Geometry check sheet. Reference: the model listing, model coordinates, mm. A direction names the side the tool comes from. Give positions to 0.01 mm unless a question says otherwise; leave off trailing zeros. Write each loop counter-clockwise with the first axis right and the second up, starting at its lowest first coordinate (ties: lowest second). Pieces come first, ordered by that corner, then holes. Notation, with made-up numbers: (37, 57.25) - (60, 57.25) arc R23 ccw to (60, 93.25) - close; hole circle Ø6 at (5.5, -4.75). An arc over 180 degrees is marked (long way). One line per question, with ' | ' between items. Start each with the question number.
Q1. Section check D-D on y = 2. Record the boundary of the cut face in (x, z), and give its area (3 significant figures).
Q2. Section check B-B on x = 172.5. Record the boundary of the cut face in (y, z).
Q3. Thickness scan on L1, parallel to X at y = -37.5, z = -74.5; L2, parallel to Z at x = 89, y = 19.5; L3, parallel to Z at x = -43, y = 19. Record the ranges inside material, lowest first. Write a range as [from, to].
Q4. Section check A-A on z = -41. Record the boundary of the cut face in (x, y).
Q5. Set-up check for faces 3 (the face through (-155.67, 36.47, -20.76)), 4 (the face through (179, 36, -74.982)), 5 (the face through (140.335, -20.881, -55.169)), 6 (the face through (-21, 37, -31.802)): record each of +Z, -Z, +X, -X, +Y, -Y from which the full face is reachable in a straight line by a thin tool's end or side.
Q6. Release check for a two-part mould opening along X. For faces 1 (the face through (-104.14, 36, -18)), 2 (the face through (3, 15, 0)) record: +X half, -X half, draft (parallel to the pull), parting line (faces both ways), or undercut.
Q7. Gauge pin test, flat ends, axial feed: P1, Ø1, axis at x = 5, z = -45, coming from the +Y side; P2, Ø9.5, axis at x = 173, z = -97.5, coming from the -Y side; P3, Ø1.5, axis at y = 32, z = -35.5, coming from the -X side; P4, Ø8.5, axis at y = -28.5, z = -69, coming from the -X side. Record the tip position at first contact, or that the pin passes through.
Q8. Section check C-C on x = -35.5. Record the boundary of the cut face in (y, z).
```python
from build123d import *

# Parameters (mm, degrees)
BOSS_EXTRUDE1_DEPTH                 = 111.76
SKETCH5_W                           = 304.8
SKETCH5_H                           = 25.4
CUT_EXTRUDE3_DEPTH                  = 101.6
CUT_EXTRUDE4_DEPTH                  = 227.288199427
CUT_EXTRUDE4_DEPTH_BACK             = 227.288199427
SKETCH3_W                           = 96.52
SKETCH3_H                           = 101.6
SKETCH3_W_2                         = 48.26
CUT_EXTRUDE5_REACH                  = 288.663
SKETCH6_W                           = 38.1
SKETCH6_H                           = 50.8
SKETCH7_W                           = 81.28
SKETCH7_H                           = 50.8
BOSS_EXTRUDE2_DEPTH                 = 5.08
SKETCH9_W                           = 5.08
SKETCH9_H                           = 95.25
BOSS_EXTRUDE3_DEPTH                 = 10.16
SKETCH10_W                          = 5.08
SKETCH10_H                          = 95.206439839
BOSS_EXTRUDE4_DEPTH                 = 10.16
CUT_EXTRUDE7_REACH                  = 208.854
FILLET1_R                           = 50.8
BOSS_EXTRUDE5_REACH                 = 208.854
CUT_EXTRUDE8_REACH                  = 248.593
CUT_EXTRUDE8_END_RADIUS             = 126.32098656
CUT_EXTRUDE8_DIRECTION_2_REACH      = 248.593
CUT_EXTRUDE8_DIRECTION_2_END_RADIUS = 126.32098656


with BuildPart() as part:
    # Sketch1 → Boss-Extrude1 (new body)
    with BuildSketch(Plane.XY):
        Polygon((-152.4, 62.23), (-152.4, -33.02), (0, -62.23), (152.4, -32.976439839), (152.4, 62.23), align=None)
    extrude(amount=-BOSS_EXTRUDE1_DEPTH)

    # Sketch5 → Cut-Extrude3 (cut)
    with BuildSketch(Plane.XY.offset(-5.08)):
        with Locations((0, -1.27)):
            Rectangle(SKETCH5_W, SKETCH5_H)
    extrude(amount=-CUT_EXTRUDE3_DEPTH, mode=Mode.SUBTRACT)

    # Sketch3 → Cut-Extrude4 (cut, two sides: drawn at the far end of the back side and taken through both)
    with BuildSketch(Plane(origin=(0, 62.23, 0), x_dir=(1, 0, 0), z_dir=(0, 1, 0)).offset(-CUT_EXTRUDE4_DEPTH_BACK)):
        with Locations((-50.8, 55.88)):
            Rectangle(SKETCH3_W, SKETCH3_H)
        with Locations((50.8, 55.88)):
            Rectangle(SKETCH3_W, SKETCH3_H)
        with Locations((-128.27, 55.88)):
            Rectangle(SKETCH3_W_2, SKETCH3_H)
        with Locations((128.27, 55.88)):
            Rectangle(SKETCH3_W_2, SKETCH3_H)
    extrude(amount=CUT_EXTRUDE4_DEPTH + CUT_EXTRUDE4_DEPTH_BACK, mode=Mode.SUBTRACT)

    # Cut-Extrude5: up to this face of the body (flat: up to its plane)
    cut_extrude5_end = Plane(part.part.faces().sort_by_distance((104.14, 36.83, -55.88))[0])
    # Sketch6 → Cut-Extrude5 (cut, up to the picked face)
    with BuildSketch(Plane.ZY.offset(104.14), mode=Mode.PRIVATE) as cut_extrude5_sk1:
        with Locations((-55.932057734, 36.83)):
            Rectangle(SKETCH6_W, SKETCH6_H)
    cut_extrude5_tool1 = split(extrude(cut_extrude5_sk1.sketch, amount=-CUT_EXTRUDE5_REACH, mode=Mode.PRIVATE), bisect_by=cut_extrude5_end, keep=Keep.BOTH, mode=Mode.PRIVATE)
    add(cut_extrude5_tool1.solids().sort_by(Axis((-104.14, 36.83, -55.932058), (1, 0, 0)))[0], mode=Mode.SUBTRACT)

    # Sketch7 → Boss-Extrude2 (add)
    with BuildSketch(Plane(origin=(0, 0, -36.882057734), x_dir=(-1, 0, 0), z_dir=(0, 0, -1))):
        with Locations((0, 36.83)):
            Rectangle(SKETCH7_W, SKETCH7_H)
        with Locations((101.6, 36.83)):
            Rectangle(SKETCH7_W, SKETCH7_H)
        with Locations((-101.6, 36.83)):
            Rectangle(SKETCH7_W, SKETCH7_H)
    boss_extrude2 = extrude(amount=-BOSS_EXTRUDE2_DEPTH)

    # Mirror1: Boss-Extrude2 across plane
    add(boss_extrude2.mirror(Plane(origin=(0, 0, -55.932057734), x_dir=(1, 0, 0), z_dir=(0, 0, -1))))

    # Sketch9 → Boss-Extrude3 (add)
    with BuildSketch(Plane.ZY.offset(152.4)):
        with Locations((-109.22, 14.605)):
            Rectangle(SKETCH9_W, SKETCH9_H)
        with Locations((-2.54, 14.605)):
            Rectangle(SKETCH9_W, SKETCH9_H)
    extrude(amount=BOSS_EXTRUDE3_DEPTH)

    # Sketch10 → Boss-Extrude4 (add)
    with BuildSketch(Plane(origin=(152.4, 0, 0), x_dir=(0, 0, -1), z_dir=(1, 0, 0))):
        with Locations((2.54, 14.626780081)):
            Rectangle(SKETCH10_W, SKETCH10_H)
        with Locations((109.22, 14.626780081)):
            Rectangle(SKETCH10_W, SKETCH10_H)
    extrude(amount=BOSS_EXTRUDE4_DEPTH)

    # Cut-Extrude7: up to this face of the body (flat: up to its plane)
    cut_extrude7_end = Plane(part.part.faces().sort_by_distance((-0.011490312, 7.400814094, -111.76))[0])
    # Sketch11 → Cut-Extrude7 (cut, up to the picked face)
    with BuildSketch(Plane.XY, mode=Mode.PRIVATE) as cut_extrude7_sk1:
        Polygon((-162.56, -12.7), (-119.696308585, -39.288207521), (-152.4, -33.02), (-162.56, -33.02), align=None)
    cut_extrude7_tool1 = split(extrude(cut_extrude7_sk1.sketch, amount=-CUT_EXTRUDE7_REACH, mode=Mode.PRIVATE), bisect_by=cut_extrude7_end, keep=Keep.BOTH, mode=Mode.PRIVATE)
    # Sketch11 → Cut-Extrude7 (cut, up to the picked face)
    with BuildSketch(Plane.XY, mode=Mode.PRIVATE) as cut_extrude7_sk2:
        Polygon((152.4, -33.02), (162.56, -33.02), (162.56, -12.7), (119.696308585, -39.288207521), align=None)
    cut_extrude7_tool2 = split(extrude(cut_extrude7_sk2.sketch, amount=-CUT_EXTRUDE7_REACH, mode=Mode.PRIVATE), bisect_by=cut_extrude7_end, keep=Keep.BOTH, mode=Mode.PRIVATE)
    add(cut_extrude7_tool1.solids().sort_by(Axis((-148.539263, -27.801749, 0), (0, 0, -1)))[0], mode=Mode.SUBTRACT)
    add(cut_extrude7_tool2.solids().sort_by(Axis((148.539263, -27.801749, 0), (0, 0, -1)))[0], mode=Mode.SUBTRACT)

    # Fillet1
    # the kernel refuses this fillet: 50.8 mm, written as the material it takes off along each edge
    with BuildSketch(Plane(origin=(-162.56, -12.7, 70.671047804), x_dir=(0.8497897447130388, -0.5271217978613181, 0), z_dir=(0, 0, -1)), Plane(origin=(-162.56, -12.7, -36.008952196), x_dir=(0.8497897447130388, -0.5271217978613181, 0), z_dir=(0, 0, -1)), Plane(origin=(162.56, -12.7, 70.671047804), x_dir=(0, 1, 0), z_dir=(0, 0, -1))) as fillet1_piece_1:
        with BuildLine():
            CenterArc((FILLET1_R * 0.556464943335, -FILLET1_R), FILLET1_R, 90, 58.188808221)
            Line((-FILLET1_R * 0.293324801378, -FILLET1_R * 0.472878202139), (0, 0))
            Line((0, 0), (FILLET1_R * 0.556464943335, 0))
        make_face()
    extrude(amount=146.422095607, mode=Mode.SUBTRACT)
    with BuildSketch(Plane(origin=(-119.696308585, -39.288207521, -83.186546401), x_dir=(0.9821230119270369, -0.18824024395268216, 0), z_dir=(0, 0, -1)), Plane(origin=(-119.696308585, -39.288207521, 23.493453599), x_dir=(0.9821230119270369, -0.18824024395268216, 0), z_dir=(0, 0, -1))) as fillet1_piece_2:
        with BuildLine():
            CenterArc((FILLET1_R * 0.184987823618, -FILLET1_R), FILLET1_R, 90, 20.961087149)
            Line((-FILLET1_R * 0.172745995297, -FILLET1_R * 0.0661764005955), (0, 0))
            Line((0, 0), (FILLET1_R * 0.184987823618, 0))
        make_face()
    extrude(amount=52.066907199, mode=Mode.SUBTRACT)
    with BuildSketch(Plane(origin=(162.56, -12.7, -36.008952196), x_dir=(-0.8497897447130388, -0.5271217978613181, 0), z_dir=(0, 0, -1))) as fillet1_piece_3:
        with BuildLine():
            CenterArc((FILLET1_R * 0.556464943335, FILLET1_R), FILLET1_R, 211.811191779, 58.188808221)
            Line((-FILLET1_R * 0.293324801378, FILLET1_R * 0.472878202139), (0, 0))
            Line((0, 0), (FILLET1_R * 0.556464943335, 0))
        make_face()
    extrude(amount=146.422095607, mode=Mode.SUBTRACT)
    with BuildSketch(Plane(origin=(119.776180176, -39.238663434, 23.475348992), x_dir=(-0.9820710795721669, -0.18851099349363817, 0), z_dir=(0, 0, -1)), Plane(origin=(119.776180176, -39.238663434, -83.204651008), x_dir=(-0.9820710795721669, -0.18851099349363817, 0), z_dir=(0, 0, -1))) as fillet1_piece_4:
        with BuildLine():
            CenterArc((FILLET1_R * 0.184845267653, FILLET1_R), FILLET1_R, 249.054708445, 20.945291555)
            Line((-FILLET1_R * 0.172631096402, FILLET1_R * 0.0660778141933), (0, 0))
            Line((0, 0), (FILLET1_R * 0.184845267653, 0))
        make_face()
    extrude(amount=52.030697984, mode=Mode.SUBTRACT)
    with BuildSketch(Plane(origin=(0, -62.23, 24.359816254), x_dir=(-0.982123011927037, 0.1882402439526816, 0), z_dir=(0, 0, -1))) as fillet1_piece_5:
        with BuildLine():
            CenterArc((FILLET1_R * 0.191809576801, FILLET1_R), FILLET1_R, 248.283995147, 21.716004853)
            Line((-FILLET1_R * 0.178196707507, FILLET1_R * 0.0709707488072), (0, 0))
            Line((0, 0), (FILLET1_R * 0.191809576801, 0))
        make_face()
    extrude(amount=160.479632508, mode=Mode.SUBTRACT)

    # Boss-Extrude5: up to this face of the body (flat: up to its plane)
    boss_extrude5_end = Plane(part.part.faces().sort_by_distance((-0.004732582, 8.379000895, -111.76))[0])
    # Sketch12 → Boss-Extrude5 (add, up to the picked face)
    with BuildSketch(Plane.XY, mode=Mode.PRIVATE) as boss_extrude5_sk1:
        with BuildLine():
            Line((-162.56, 62.23), (-210.82, 62.23))
            ThreePointArc((-210.82, 62.23), (-185.525923559, 8.586514121), (-138.537787331, -27.60089991))
            Line((-138.537787331, -27.60089991), (-162.56, 62.23))
        make_face()
    boss_extrude5_tool1 = split(extrude(boss_extrude5_sk1.sketch, amount=-BOSS_EXTRUDE5_REACH, mode=Mode.PRIVATE), bisect_by=boss_extrude5_end, keep=Keep.BOTH, mode=Mode.PRIVATE)
    # Sketch12 → Boss-Extrude5 (add, up to the picked face)
    with BuildSketch(Plane.XY, mode=Mode.PRIVATE) as boss_extrude5_sk2:
        with BuildLine():
            Line((162.56, 62.23), (210.82, 62.23))
            ThreePointArc((210.82, 62.23), (185.525923559, 8.586514121), (138.537787331, -27.60089991))
            Line((138.537787331, -27.60089991), (162.56, 62.23))
        make_face()
    boss_extrude5_tool2 = split(extrude(boss_extrude5_sk2.sketch, amount=-BOSS_EXTRUDE5_REACH, mode=Mode.PRIVATE), bisect_by=boss_extrude5_end, keep=Keep.BOTH, mode=Mode.PRIVATE)
    add(boss_extrude5_tool1.solids().sort_by(Axis((-173.436994, 26.131053, 0), (0, 0, -1)))[0])
    add(boss_extrude5_tool2.solids().sort_by(Axis((173.436994, 26.131053, 0), (0, 0, -1)))[0])

    # Cut-Extrude8: up to this cylinder (the profile starts inside it)
    cut_extrude8_end = Plane(origin=(-87.109319049, 87.777192878, -55.90231), z_dir=(0, 0, 1)) * Cylinder(CUT_EXTRUDE8_END_RADIUS, 750.827973119, mode=Mode.PRIVATE)
    # Sketch13 → Cut-Extrude8 (cut, up to the surface)
    with BuildSketch(Plane(origin=(0, 0, 0), x_dir=(0, 0, -1), z_dir=(1, 0, 0)), mode=Mode.PRIVATE) as cut_extrude8_sk1:
        Polygon((36.882057734, 62.23), (36.882057734, 11.43), (5.08, 11.43), (5.08, -13.97), (106.68, -13.97), (106.68, 11.43), (74.982057734, 11.43), (74.982057734, 62.23), align=None)
    cut_extrude8_tool1 = extrude(cut_extrude8_sk1.sketch, amount=-CUT_EXTRUDE8_REACH, mode=Mode.PRIVATE) & cut_extrude8_end
    add(cut_extrude8_tool1.solids().sort_by_distance((0, 15.058571, -55.90231))[0], mode=Mode.SUBTRACT)

    # Cut-Extrude8 direction 2: up to this cylinder (the profile starts inside it)
    cut_extrude8_direction_2_end = Plane(origin=(87.109319049, 87.777192878, -55.90231), z_dir=(0, 0, 1)) * Cylinder(CUT_EXTRUDE8_DIRECTION_2_END_RADIUS, 750.827973119, mode=Mode.PRIVATE)
    # Sketch13 → Cut-Extrude8 direction 2 (cut, up to the surface)
    with BuildSketch(Plane(origin=(0, 0, 0), x_dir=(0, 0, -1), z_dir=(1, 0, 0)), mode=Mode.PRIVATE) as cut_extrude8_direction_2_sk1:
        Polygon((36.882057734, 62.23), (36.882057734, 11.43), (5.08, 11.43), (5.08, -13.97), (106.68, -13.97), (106.68, 11.43), (74.982057734, 11.43), (74.982057734, 62.23), align=None)
    cut_extrude8_direction_2_tool1 = extrude(cut_extrude8_direction_2_sk1.sketch, amount=CUT_EXTRUDE8_DIRECTION_2_REACH, mode=Mode.PRIVATE) & cut_extrude8_direction_2_end
    add(cut_extrude8_direction_2_tool1.solids().sort_by_distance((0, 15.058571, -55.90231))[0], mode=Mode.SUBTRACT)


solid = part.part
```
Working result:
1) outline: (-179.84, -111.76) - (179.84, -111.76) - (179.84, -106.68) - (-179.84, -106.68) - close; (-179.84, -5.08) - (179.84, -5.08) - (179.84, 0) - (-179.84, 0) - close | area: 3,650 mm2
2) outline: (-5.31, -111.76) - (62.23, -111.76) - (62.23, -74.98) - (11.43, -74.98) - (11.43, -106.68) - (-5.31, -106.68) - close; (-5.31, -5.08) - (11.43, -5.08) - (11.43, -36.88) - (62.23, -36.88) - (62.23, 0) - (-5.31, 0) - close
3) L1: x = [-104.14, -99.06], [-2.54, 2.54], [99.06, 104.14] | L2: z = [-111.76, -106.68], [-80.06, -74.98], [-36.88, -31.8], [-5.08, 0] | L3: z = [-111.76, -106.68], [-5.08, 0]
4) outline: (-161.97, -13.97) arc R126.32 ccw to (-138.54, -27.6) - (-142.18, -13.97) - close; (-104.14, -42.27) - (-99.06, -43.24) - (-99.06, -13.97) - (-104.14, -13.97) - close; (-2.54, -61.24) arc R50.8 ccw to (2.54, -61.24) - (2.54, -13.97) - (-2.54, -13.97) - close; (99.06, -43.22) - (104.14, -42.24) - (104.14, -13.97) - (99.06, -13.97) - close; (138.54, -27.6) arc R126.32 ccw to (161.97, -13.97) - (142.18, -13.97) - close
5) face 3: +Y | face 4: +X, -X, +Y | face 5: none | face 6: +Y, -Y
6) face 1: undercut | face 2: draft
7) P1: passes through | P2: stops at y = 11.43 | P3: stops at x = -200.82 | P4: stops at x = -145.48
8) outline: (-55.43, -111.76) - (62.23, -111.76) - (62.23, -106.68) - (-55.43, -106.68) - close; (-55.43, -5.08) - (62.23, -5.08) - (62.23, 0) - (-55.43, 0) - close; (11.43, -80.06) - (62.23, -80.06) - (62.23, -74.98) - (11.43, -74.98) - close; (11.43, -36.88) - (62.23, -36.88) - (62.23, -31.8) - (11.43, -31.8) - close
